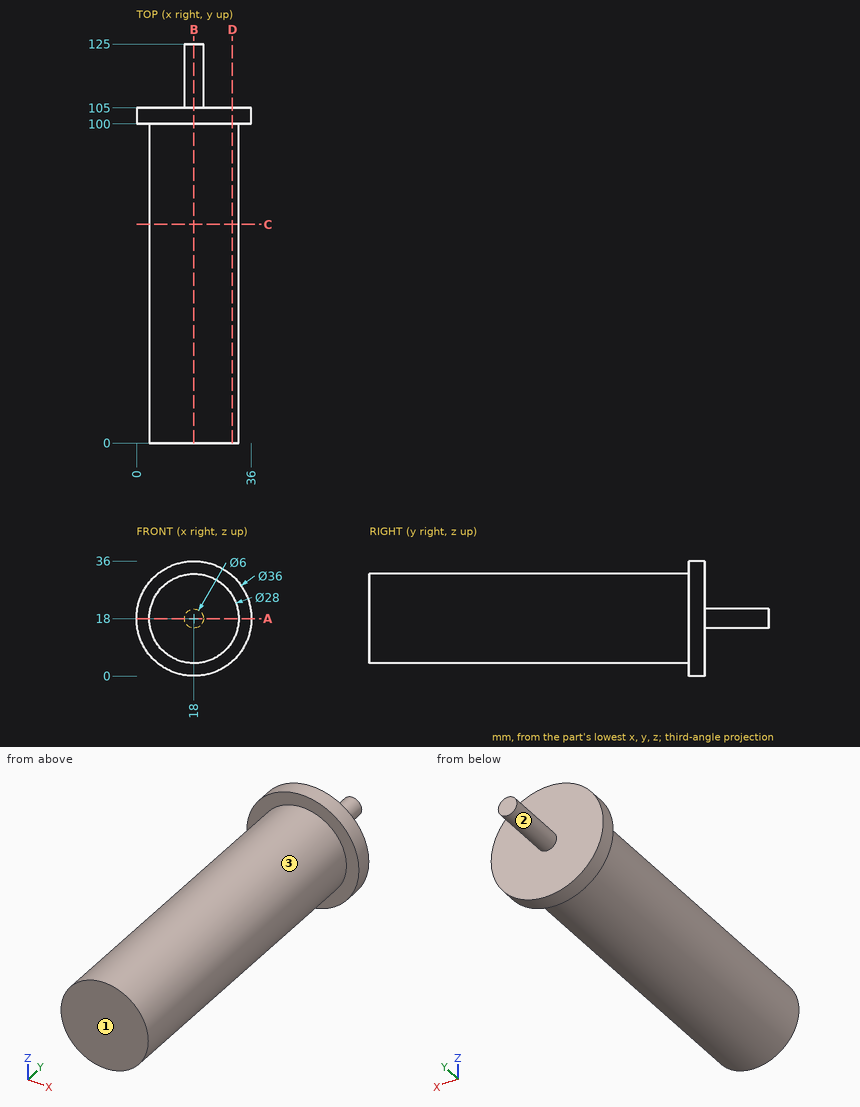
Geometry: see drawing. Coordinates: mm, zero at the bounding-box minimum. A direction names the side the tool comes from. Give positions to 0.01 mm unless a question says otherwise; leave off trailing zeros. Loops run counter-clockwise (first coordinate to the right, second up) from the corner with the lowest first, then second, coordinate; pieces in that order, holes last. Notation, with made-up numbers: (58, 71.5) - (91, 71.5) arc R15 cw to (91, 87.5) - close; hole circle Ø5 at (81, 24). An arc over 180 degrees is marked (long way). Use CSV: the item, a comma, the result in double quotes. Start each with the question number.
1. Section B-B (x = 18). Output: boundary loops of the cut face in (y, z), then the cut area to 3 significant figures.
2. Ray query, L1, parallel to Y at x = 11, z = 31; L2, parallel to Z at x = 17.5, y = 87; L3, parallel to Y at x = 13, z = 23.5. Return the intervals inside material, ascending.
3. Reachability of the marked faces 1, 2 and 3 from +Z, -Z, +X, -X, +Y, -Y: full face, straight path, thin tool, end or side. Return the list, or none.
4. Section D-D (x = 30). Output: boundary loops of the cut face in (y, z), then the cut area to 3 significant figures.
5. Pin query (flat end, axial travel): pin 1 (12 mm diameter, centred on x = 22, y = 104, fed in from -Z); pin 2 (5 mm diameter, centred on y = 17.5, z = 12.5, fed in from +X); pin 3 (2 mm diameter, centred on y = 58, z = 18, fed in from +X); pin 4 (1.5 mm diameter, centred on x = 8.5, y = 107, fed in from -Z). Return the tip coordinate at first contact, or that it passes through.
6. Section A-A (z = 18). Output: boundary loops of the cut face in (x, y).
7. Section C-C (y = 68.5). Output: boundary loops of the cut face in (x, z), then the cut area to 3 significant figures.
Response:
1,outline,"(0, 4) - (100, 4) - (100, 0) - (105, 0) - (105, 15) - (125, 15) - (125, 21) - (105, 21) - (105, 36) - (100, 36) - (100, 32) - (0, 32) - close"
1,area,"3,100 mm²"
2,L1,"100 to 105"
2,L2,"4.01 to 31.99"
2,L3,"0 to 105"
3,face 1,"+Z, -Z, +X, -X, -Y"
3,face 2,"+Y"
3,face 3,"-Y"
4,outline,"(0, 10.79) - (100, 10.79) - (100, 4.58) - (105, 4.58) - (105, 31.42) - (100, 31.42) - (100, 25.21) - (0, 25.21) - close"
4,area,"1,580 mm²"
5,pin 1,"z = 0"
5,pin 2,"x = 31.67"
5,pin 3,"x = 32"
5,pin 4,"through"
6,outline,"(0, 100) - (4, 100) - (4, 0) - (32, 0) - (32, 100) - (36, 100) - (36, 105) - (21, 105) - (21, 125) - (15, 125) - (15, 105) - (0, 105) - close"
7,outline,"circle Ø28 at (18, 18)"
7,area,"616 mm²"
